```python
from build123d import *

# Parameters (mm, degrees)
F1_DEPTH = 3.175
F3_DEPTH = 1.5875
F5_DEPTH = 3.175
F7_DEPTH = 3.175


with BuildPart() as f1:
    # F0 (on Top) → F1 (new body)
    with BuildSketch(Plane.XY):
        Polygon((0, 266.7), (-38.1, 215.9), (-19.05, -266.7), (19.05, -266.7), (38.1, 215.9), align=None)
    extrude(amount=F1_DEPTH)

    # F2 (on Top) → F3 (cut)
    with BuildSketch(Plane.XY):
        Polygon((31.745055, 215.9), (-31.745055, 215.9), (-12.685168, -266.950463), (-9.512639, -266.825231), (-28.316924, 209.55), (28.316924, 209.55), (9.517582, -266.7), (12.690111, -266.825231), align=None)
    extrude(amount=F3_DEPTH, mode=Mode.SUBTRACT)

    # F4 (on face) → F5 (cut)
    with BuildSketch(Plane.XY.offset(3.175)):
        Polygon((31.745055, 215.9), (-31.745055, 215.9), (-31.494397, 209.55), (31.494397, 209.55), align=None)
    extrude(amount=-F5_DEPTH, mode=Mode.SUBTRACT)

    # F6 (on face) → F7 (join)
    with BuildSketch(Plane(origin=(0, 0, 0), x_dir=(1, 0, 0), z_dir=(0, 0, -1))):
        Polygon((-19.05, 266.7), (-38.1, -215.9), (0, -266.7), (38.1, -215.9), (19.05, 266.7), align=None)
    extrude(amount=F7_DEPTH)


solid = f1.part
```
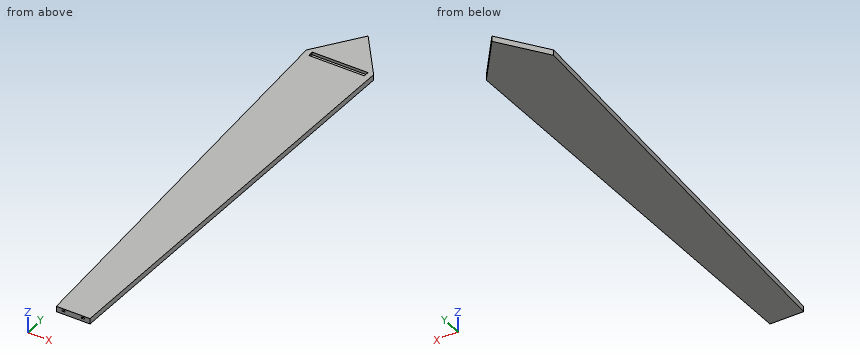
For this review, take the finished solid that the model builds, in its own axes (mm). Round coordinates to 2 decimals unless told otherwise and drop trailing zeros. Write each loop counter-clockwise with the first axis right and the second up, starting at its lowest first coordinate (ties: lowest second). Pieces come first, ordered by that corner, then holes. Notation, with made-up numbers: M -29.5,80 L -21.5,80 A17 ccw -21.5,112 Z; hole C -23,-5 d11. An arc over 180 degrees is marked long. One line per item, written item: value. Start each with the question number.
(1) Insertion check: pin 1 (1 mm diameter, centred on x = 15.5, z = 1.5, fed in from +Y); pin 2 (2 mm diameter, centred on y = -20.5, z = 1, fed in from +X); pin 3 (2 mm diameter, centred on x = 28, z = 0, fed in from +Y). Each pin has a flat end and moves straight along its axis. Give the tip position at first contact, or say it passes through.
(2) We need section B-B (z = -2). Give the boundary of the cut face in (x, y).
(3) Wall thickness on line 1 (X direction, y = -44.5, z = 1.25); line 2 (Z direction, x = -17.5, y = -96) (1 decimal); line 3 (Y direction, x = 19, z = 2.25): over which ranges is each line inside the solid? List them lowest first.
(4) We need section A-A (y = -165.5). Give the boundary of the cut face in (x, z) (1 decimal), and give its area (3 significant figures).
(5) We need section C-C (y = -55). Give the boundary of the cut face in (x, z) (1 decimal), and give its area (3 significant figures).
Result:
1. pin 1: y = 246.7
1. pin 2: x = 28.81
1. pin 3: y = 230.7
2. outline: M -38.1,215.9 L -19.05,-266.7 L 19.05,-266.7 L 38.1,215.9 L 0,266.7 Z
3. line 1: -27.82 to -21.47, -18.29 to 18.29, 21.47 to 27.82
3. line 2: -3.2 to 0, 1.6 to 3.2
3. line 3: -266.7 to 209.55, 215.9 to 241.37
4. outline: M -23,-3.2 L 23,-3.2 L 23,3.2 L -23,3.2 Z; hole M -16.7,0 L -13.5,0 L -13.5,1.6 L -16.7,1.6 Z; hole M 13.5,0 L 16.7,0 L 16.7,1.6 L 13.5,1.6 Z
4. area: 283 mm²
5. outline: M -27.4,-3.2 L 27.4,-3.2 L 27.4,3.2 L -27.4,3.2 Z; hole M -21.1,0 L -17.9,0 L -17.9,1.6 L -21.1,1.6 Z; hole M 17.9,0 L 21.1,0 L 21.1,1.6 L 17.9,1.6 Z
5. area: 338 mm²
